```python
from build123d import *

# Parameters (mm, degrees)
SKETCH_3_R                      = 1.7
CUT_EXTRUDE_1_DEPTH             = 10
CUT_EXTRUDE_1_DIRECTION_2_REACH = 60.902
CUT_EXTRUDE_START               = 3
SKETCH_4_R                      = 3
CUT_EXTRUDE_2_DEPTH             = 3
SKETCH_7_R                      = 3
CUT_EXTRUDE_3_DEPTH             = 10
EXTRUDE_1_DEPTH                 = 1


# Read off the part's stored shape, not the designer's step: the extrude step
with BuildPart() as part:
    # Sketch 2 → Revolve 1 (revolve)
    with BuildSketch(Plane(origin=(0, 0, 0), x_dir=(0, 0, -1), z_dir=(1, 0, 0)), mode=Mode.PRIVATE) as revolve_1_sk:
        Polygon((-30, 0), (-30, 2), (-36, 2), (-36, -1.5), (-41.5, -1.5), (-41.5, -6.5), (-35, -6.5), (-35, -5.5), (-33.5, -5.5), (-33.5, 0), align=None)
    revolve(revolve_1_sk.sketch.rotate(Axis((0, 0, 0), (0, 1, 0)), 180), axis=Axis((0, 0, 0), (0, 1, 0)))

    # Sketch 3 → Cut-Extrude 1 (cut)
    with BuildSketch(Plane(origin=(0, -1.5, 0), x_dir=(1, 0, 0), z_dir=(0, 1, 0))):
        with Locations(Location((0, 37, 0), (0, 0, 217.103674805))):
            Circle(SKETCH_3_R)
        with Locations(Location((32.04293994, 18.5, 0), (0, 0, 157.103674805))):
            Circle(SKETCH_3_R)
        with Locations(Location((32.04293994, -18.5, 0), (0, 0, 97.103674805))):
            Circle(SKETCH_3_R)
        with Locations(Location((0, -37, 0), (0, 0, 37.103674804))):
            Circle(SKETCH_3_R)
        with Locations(Location((-32.04293994, -18.5, 0), (0, 0, 82.896325196))):
            Circle(SKETCH_3_R)
        with Locations(Location((-32.04293994, 18.5, 0), (0, 0, 22.896325196))):
            Circle(SKETCH_3_R)
    extrude(amount=-CUT_EXTRUDE_1_DEPTH, mode=Mode.SUBTRACT)

    # Sketch 3 → Cut-Extrude 1 direction 2 (cut, up to next)
    with BuildSketch(Plane(origin=(0, -1.5, 0), x_dir=(1, 0, 0), z_dir=(0, 1, 0)), mode=Mode.PRIVATE) as cut_extrude_1_direction_2_sk1:
        with Locations(Location((0, 37, 0), (0, 0, 217.103674805))):
            Circle(SKETCH_3_R)
    cut_extrude_1_direction_2_tool1 = extrude(cut_extrude_1_direction_2_sk1.sketch, amount=CUT_EXTRUDE_1_DIRECTION_2_REACH, mode=Mode.PRIVATE) & part.part
    # Sketch 3 → Cut-Extrude 1 direction 2 (cut, up to next)
    with BuildSketch(Plane(origin=(0, -1.5, 0), x_dir=(1, 0, 0), z_dir=(0, 1, 0)), mode=Mode.PRIVATE) as cut_extrude_1_direction_2_sk2:
        with Locations(Location((32.04293994, 18.5, 0), (0, 0, 157.103674805))):
            Circle(SKETCH_3_R)
    cut_extrude_1_direction_2_tool2 = extrude(cut_extrude_1_direction_2_sk2.sketch, amount=CUT_EXTRUDE_1_DIRECTION_2_REACH, mode=Mode.PRIVATE) & part.part
    # Sketch 3 → Cut-Extrude 1 direction 2 (cut, up to next)
    with BuildSketch(Plane(origin=(0, -1.5, 0), x_dir=(1, 0, 0), z_dir=(0, 1, 0)), mode=Mode.PRIVATE) as cut_extrude_1_direction_2_sk3:
        with Locations(Location((32.04293994, -18.5, 0), (0, 0, 97.103674805))):
            Circle(SKETCH_3_R)
    cut_extrude_1_direction_2_tool3 = extrude(cut_extrude_1_direction_2_sk3.sketch, amount=CUT_EXTRUDE_1_DIRECTION_2_REACH, mode=Mode.PRIVATE) & part.part
    # Sketch 3 → Cut-Extrude 1 direction 2 (cut, up to next)
    with BuildSketch(Plane(origin=(0, -1.5, 0), x_dir=(1, 0, 0), z_dir=(0, 1, 0)), mode=Mode.PRIVATE) as cut_extrude_1_direction_2_sk4:
        with Locations(Location((0, -37, 0), (0, 0, 37.103674804))):
            Circle(SKETCH_3_R)
    cut_extrude_1_direction_2_tool4 = extrude(cut_extrude_1_direction_2_sk4.sketch, amount=CUT_EXTRUDE_1_DIRECTION_2_REACH, mode=Mode.PRIVATE) & part.part
    # Sketch 3 → Cut-Extrude 1 direction 2 (cut, up to next)
    with BuildSketch(Plane(origin=(0, -1.5, 0), x_dir=(1, 0, 0), z_dir=(0, 1, 0)), mode=Mode.PRIVATE) as cut_extrude_1_direction_2_sk5:
        with Locations(Location((-32.04293994, -18.5, 0), (0, 0, 82.896325196))):
            Circle(SKETCH_3_R)
    cut_extrude_1_direction_2_tool5 = extrude(cut_extrude_1_direction_2_sk5.sketch, amount=CUT_EXTRUDE_1_DIRECTION_2_REACH, mode=Mode.PRIVATE) & part.part
    # Sketch 3 → Cut-Extrude 1 direction 2 (cut, up to next)
    with BuildSketch(Plane(origin=(0, -1.5, 0), x_dir=(1, 0, 0), z_dir=(0, 1, 0)), mode=Mode.PRIVATE) as cut_extrude_1_direction_2_sk6:
        with Locations(Location((-32.04293994, 18.5, 0), (0, 0, 22.896325196))):
            Circle(SKETCH_3_R)
    cut_extrude_1_direction_2_tool6 = extrude(cut_extrude_1_direction_2_sk6.sketch, amount=CUT_EXTRUDE_1_DIRECTION_2_REACH, mode=Mode.PRIVATE) & part.part
    add(cut_extrude_1_direction_2_tool1.solids().sort_by_distance((0, -1.5, -37))[0], mode=Mode.SUBTRACT)
    add(cut_extrude_1_direction_2_tool2.solids().sort_by_distance((32.04294, -1.5, -18.5))[0], mode=Mode.SUBTRACT)
    add(cut_extrude_1_direction_2_tool3.solids().sort_by_distance((32.04294, -1.5, 18.5))[0], mode=Mode.SUBTRACT)
    add(cut_extrude_1_direction_2_tool4.solids().sort_by_distance((0, -1.5, 37))[0], mode=Mode.SUBTRACT)
    add(cut_extrude_1_direction_2_tool5.solids().sort_by_distance((-32.04294, -1.5, 18.5))[0], mode=Mode.SUBTRACT)
    add(cut_extrude_1_direction_2_tool6.solids().sort_by_distance((-32.04294, -1.5, -18.5))[0], mode=Mode.SUBTRACT)

    # Sketch 4 → Cut-Extrude 2 (cut)
    with BuildSketch(Plane(origin=(0, -1.5, 0), x_dir=(1, 0, 0), z_dir=(0, 1, 0)).offset(CUT_EXTRUDE_START)):
        with Locations((0, 37)):
            Circle(SKETCH_4_R)
        with Locations((32.04293994, 18.5)):
            Circle(SKETCH_4_R)
        with Locations((32.04293994, -18.5)):
            Circle(SKETCH_4_R)
        with Locations((0, -37)):
            Circle(SKETCH_4_R)
        with Locations((-32.04293994, -18.5)):
            Circle(SKETCH_4_R)
        with Locations((-32.04293994, 18.5)):
            Circle(SKETCH_4_R)
    extrude(amount=CUT_EXTRUDE_2_DEPTH, mode=Mode.SUBTRACT)

    # Sketch 7 → Cut-Extrude 3 (cut)
    with BuildSketch(Plane(origin=(0, -1.5, 0), x_dir=(1, 0, 0), z_dir=(0, 1, 0))):
        with Locations((32.04293994, 18.5)):
            Circle(SKETCH_7_R)
    extrude(amount=CUT_EXTRUDE_3_DEPTH, mode=Mode.SUBTRACT)

    # Extrude 1 outline → Extrude 1 (add)
    with BuildSketch(Plane(origin=(0, -1.5, 0), x_dir=(1, 0, 0), z_dir=(0, 1, 0))):
        with BuildLine():
            ThreePointArc((31.832709232, 16.813049186), (30.570696753, 17.65), (30.476882326, 19.161410274))
            ThreePointArc((30.476882326, 19.161410274), (30.089095942, 19.764774357), (29.689366173, 20.360293128))
            ThreePointArc((29.689366173, 20.360293128), (29.444863729, 17), (32.477214164, 15.531598764))
            ThreePointArc((32.477214164, 15.531598764), (32.161344664, 16.175534285), (31.832709232, 16.813049186))
        make_face()
    extrude(amount=EXTRUDE_1_DEPTH)


solid = part.part
```
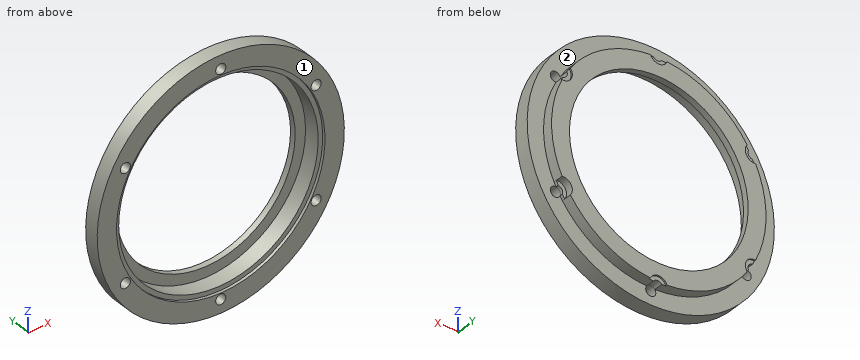
Build history of the part. All positions in model axes, mm. Face numbers are marked on the shaded views. A direction names the side the tool comes from. Round coordinates to 2 decimals unless told otherwise and drop trailing zeros. Loops run counter-clockwise (first coordinate to the right, second up) from the corner with the lowest first, then second, coordinate; pieces in that order, holes last. Notation, with made-up numbers: M 82,13 L 120,13 A30 ccw 120,38 Z; hole C -25.75,58 d9. An arc over 180 degrees is marked long. Answer as CSV lines item,"result".
1. Wall check: probe 1 along X at (y, z) = (-3.75, 18.5); probe 2 along X at (y, z) = (-2, -17); probe 3 along X at (y, z) = (-6.2, 0). Give the ranges that are in metal, low to high. Write a range as [from, to].
Resolved:
probe 1,"x = [-37.15, -33.74], [-30.34, -27.93], [27.93, 30.34], [33.74, 37.15]"
probe 2,"x = [-37.86, -32.84], [-31.24, -28.87], [28.87, 31.24], [32.84, 37.86]"
probe 3,"x = [-41.5, -35], [35, 41.5]"
2. Cut at D-D on x = -28. Write the cut outline in (y, z), then the cut area to 3 significant figures.
Resolved:
outline,"M -6.5,-30.63 L -1.5,-30.63 L -1.5,-22.63 L 2,-22.63 L 2,-10.77 L 0,-10.77 L 0,-18.39 L -5.5,-18.39 L -5.5,-21 L -6.5,-21 Z; M -6.5,21 L -5.5,21 L -5.5,18.39 L 0,18.39 L 0,10.77 L 2,10.77 L 2,22.63 L -1.5,22.63 L -1.5,30.63 L -6.5,30.63 Z"
area,"177 mm²"
3. Cut at C-C on y = -2.75. Write the cut outline in (x, z), then the cut area to 3 significant figures.
Resolved:
outline,"C 0,0 d83; hole C -32.04,-18.5 d3.4; hole C -32.04,18.5 d3.4; hole C 0,0 d67; hole C 0,-37 d3.4; hole C 0,37 d3.4; hole C 32.04,-18.5 d3.4; hole C 32.04,18.5 d3.4"
area,"1,830 mm²"
4. Cut at A-A on z = 0. Write the cut outline in (x, y).
Resolved:
outline,"M -41.5,-6.5 L -35,-6.5 L -35,-5.5 L -33.5,-5.5 L -33.5,0 L -30,0 L -30,2 L -36,2 L -36,-1.5 L -41.5,-1.5 Z; M 30,0 L 33.5,0 L 33.5,-5.5 L 35,-5.5 L 35,-6.5 L 41.5,-6.5 L 41.5,-1.5 L 36,-1.5 L 36,2 L 30,2 Z"
5. Flat gauge pins, fed straight in: P1, Ø4, axis at x = -32.04, z = 18.5, coming from the -Y side; P2, Ø20, axis at x = 9, z = -11, coming from the -Y side; P3, Ø1, axis at x = -4.5, y = -4.5, coming from the +Z side; P4, Ø1.7, axis at x = 30.5, z = 19, coming from the +Y side. Where does each tip first touch, or does it go through?
Resolved:
P1,"stops at y = -6.5"
P2,"passes through"
P3,"stops at z = 41.31"
P4,"stops at y = 1.5"
6. 3-axis set-ups, long thin cutter, end or side, ignore diameter. For the marked faces 1 and 2: which of +Z, -Z, +X, -X, +Y, -Y reach the whole face in a straight line?
Resolved:
face 1,"+Z, -Z, +X, -X, -Y"
face 2,"+Y"
7. Cut at B-B on x = 0. Write the cut outline in (y, z).
Resolved:
outline,"M -6.5,-41.5 L -1.5,-41.5 L -1.5,-38.7 L -6.5,-38.7 Z; M -6.5,-35.3 L 1.5,-35.3 L 1.5,-34 L 2,-34 L 2,-30 L 0,-30 L 0,-33.5 L -5.5,-33.5 L -5.5,-35 L -6.5,-35 Z; M -6.5,35 L -5.5,35 L -5.5,33.5 L 0,33.5 L 0,30 L 2,30 L 2,34 L 1.5,34 L 1.5,35.3 L -6.5,35.3 Z; M -6.5,38.7 L -1.5,38.7 L -1.5,41.5 L -6.5,41.5 Z"
